from build123d import *

# Parameters (mm, degrees)
F0_W           = 30
F0_H           = 30
F0_R           = 4
F1_DEPTH       = 11
F3_D           = 3.4
F3_CBORE_D     = 6.3
F3_CBORE_DEPTH = 8.5
F5_D           = 3.4
F6_DEPTH       = 5
F7_R           = 4
F8_DEPTH       = 7
F9_R           = 5
F10_T1_DEPTH   = 9.5
F10_T3_DEPTH   = 20
F10_T5_DEPTH   = 20
F10_T12_ANGLE  = 90
F10_T14_ANGLE  = 90
F10_T16_ANGLE  = 90
F10_T18_ANGLE  = 90


# Not quite as in the source:
# - a fillet or chamfer that OpenCascade refuses, or shapes differently, is made with other operations: its cross-section is extruded or revolved along the edge and cut away or added


with BuildPart() as f1:
    # F0 (on Top) → F1 (new body)
    with BuildSketch(Plane.XY):
        Rectangle(F0_W, F0_H)
        Circle(F0_R, mode=Mode.SUBTRACT)
    extrude(amount=F1_DEPTH)

    # F3 (through all)
    with Locations(Plane.XY.offset(11)):
        with Locations((-6.7175144213, -6.7175144213), (-5.6568542495, 5.6568542495), (6.7175144213, 6.7175144213), (5.6568542495, -5.6568542495)):
            CounterBoreHole(F3_D / 2, F3_CBORE_D / 2, F3_CBORE_DEPTH)

    # F5 (through all)
    with Locations(Plane(origin=(0, 0, 0), x_dir=(1, 0, 0), z_dir=(0, 0, -1))):
        with Locations((-11, 0), (11, 0)):
            Hole(F5_D / 2)

    # F4 (on face) → F6 (cut)
    with BuildSketch(Plane(origin=(0, 0, 0), x_dir=(1, 0, 0), z_dir=(0, 0, -1))):
        Polygon((14, -1.7320508076), (14, 1.7320508076), (11, 3.4641016151), (8, 1.7320508076), (8, -1.7320508076), (11, -3.4641016151), align=None)
        Polygon((-8, -1.7320508076), (-8, 1.7320508076), (-11, 3.4641016151), (-14, 1.7320508076), (-14, -1.7320508076), (-11, -3.4641016151), align=None)
    extrude(amount=-F6_DEPTH, mode=Mode.SUBTRACT)

    # F7 (on face) → F8 (cut)
    with BuildSketch(Plane.XY.offset(11)):
        with BuildLine():
            Line((-7.75, -15), (7.75, -15))
            Line((7.75, -15), (7.75, -8.0108382909))
            ThreePointArc((7.75, -8.0108382909), (2.5068542495, -5.6568542495), (7.75, -3.3028702081))
            Line((7.75, -3.3028702081), (7.75, 3.7415316374))
            ThreePointArc((7.75, 3.7415316374), (3.5675144213, 6.7175144213), (7.75, 9.6934972051))
            Line((7.75, 9.6934972051), (7.75, 15))
            Line((7.75, 15), (-7.75, 15))
            Line((-7.75, 15), (-7.75, 8.0108382909))
            ThreePointArc((-7.75, 8.0108382909), (-4.3666816087, 8.5305199498), (-2.5068542495, 5.6568542495))
            ThreePointArc((-2.5068542495, 5.6568542495), (-4.3666816087, 2.7831885492), (-7.75, 3.3028702081))
            Line((-7.75, 3.3028702081), (-7.75, -3.7415316374))
            ThreePointArc((-7.75, -3.7415316374), (-4.8912928538, -4.1509184682), (-3.5675144213, -6.7175144213))
            ThreePointArc((-3.5675144213, -6.7175144213), (-4.8912928538, -9.2841103744), (-7.75, -9.6934972051))
            Line((-7.75, -9.6934972051), (-7.75, -15))
        make_face()
        Circle(F7_R, mode=Mode.SUBTRACT)
    extrude(amount=-F8_DEPTH, mode=Mode.SUBTRACT)

    # F9
    f9_edges = [f1.edges().sort_by_distance(p)[0] for p in [
        (15, 15, 5.5),
        (-15, 15, 5.5),
        (15, -15, 5.5),
        (-15, -15, 5.5),
    ]]
    fillet(f9_edges, radius=F9_R)

    # F10: fillet of radius 1 on 15 edges, made by hand

    # F10_s2 → F10_t1 (cut)
    with BuildSketch(Plane.XY.offset(4)):
        with BuildLine():
            ThreePointArc((8.75, 15), (8.0428932188, 14.7071067812), (7.75, 14))
            Line((7.75, 14), (7.75, 15))
            Line((7.75, 15), (8.75, 15))
        make_face()
        with BuildLine():
            ThreePointArc((-8.75, 15), (-8.0428932188, 14.7071067812), (-7.75, 14))
            Line((-7.75, 14), (-7.75, 15))
            Line((-7.75, 15), (-8.75, 15))
        make_face()
        with BuildLine():
            ThreePointArc((8.75, -15), (8.0428932188, -14.7071067812), (7.75, -14))
            Line((7.75, -14), (7.75, -15))
            Line((7.75, -15), (8.75, -15))
        make_face()
        with BuildLine():
            ThreePointArc((-8.75, -15), (-8.0428932188, -14.7071067812), (-7.75, -14))
            Line((-7.75, -14), (-7.75, -15))
            Line((-7.75, -15), (-8.75, -15))
        make_face()
    extrude(amount=F10_T1_DEPTH, mode=Mode.SUBTRACT)

    # F10_s4 → F10_t3 (cut)
    with BuildSketch(Plane.YZ.offset(-10)):
        with BuildLine():
            ThreePointArc((-15, 1), (-14.7071067812, 0.2928932188), (-14, 0))
            Line((-14, 0), (-15, 0))
            Line((-15, 0), (-15, 1))
        make_face()
        with BuildLine():
            ThreePointArc((14, 0), (14.7071067812, 0.2928932188), (15, 1))
            Line((15, 1), (15, 0))
            Line((15, 0), (14, 0))
        make_face()
    extrude(amount=F10_T3_DEPTH, mode=Mode.SUBTRACT)

    # F10_s6 → F10_t5 (cut)
    with BuildSketch(Plane.XZ.offset(-10)):
        with BuildLine():
            ThreePointArc((-14, 0), (-14.7071067812, 0.2928932188), (-15, 1))
            Line((-15, 1), (-15, 0))
            Line((-15, 0), (-14, 0))
        make_face()
        with BuildLine():
            ThreePointArc((14, 0), (14.7071067812, 0.2928932188), (15, 1))
            Line((15, 1), (15, 0))
            Line((15, 0), (14, 0))
        make_face()
    extrude(amount=F10_T5_DEPTH, mode=Mode.SUBTRACT)

    # F10_s7 → F10_t8 (revolve, cut)
    with BuildSketch(Plane.XZ):
        with BuildLine():
            ThreePointArc((5, 4), (4.2928932188, 3.7071067812), (4, 3))
            Line((4, 3), (4, 4))
            Line((4, 4), (5, 4))
        make_face()
    revolve(axis=Axis((0, 0, 4), (0, 0, 1)), mode=Mode.SUBTRACT)

    # F10_s9 → F10_t10 (revolve, cut)
    with BuildSketch(Plane.XZ):
        with BuildLine():
            ThreePointArc((5, 0), (4.2928932188, 0.2928932188), (4, 1))
            Line((4, 1), (4, 0))
            Line((4, 0), (5, 0))
        make_face()
    revolve(axis=Axis((0, 0, 0), (0, 0, 1)), mode=Mode.SUBTRACT)

    # F10_s11 → F10_t12 (revolve, cut)
    with BuildSketch(Plane.YZ.offset(-10)):
        with BuildLine():
            ThreePointArc((-14, 0), (-14.7071067812, 0.2928932188), (-15, 1))
            Line((-15, 1), (-15, 0))
            Line((-15, 0), (-14, 0))
        make_face()
    revolve(axis=Axis((-10, -10, 0), (0, 0, -1)), revolution_arc=F10_T12_ANGLE, mode=Mode.SUBTRACT)

    # F10_s13 → F10_t14 (revolve, cut)
    with BuildSketch(Plane.YZ.offset(10)):
        with BuildLine():
            ThreePointArc((-14, 0), (-14.7071067812, 0.2928932188), (-15, 1))
            Line((-15, 1), (-15, 0))
            Line((-15, 0), (-14, 0))
        make_face()
    revolve(axis=Axis((10, -10, 0), (0, 0, 1)), revolution_arc=F10_T14_ANGLE, mode=Mode.SUBTRACT)

    # F10_s15 → F10_t16 (revolve, cut)
    with BuildSketch(Plane.XZ.offset(-10)):
        with BuildLine():
            ThreePointArc((-14, 0), (-14.7071067812, 0.2928932188), (-15, 1))
            Line((-15, 1), (-15, 0))
            Line((-15, 0), (-14, 0))
        make_face()
    revolve(axis=Axis((-10, 10, 0), (0, 0, -1)), revolution_arc=F10_T16_ANGLE, mode=Mode.SUBTRACT)

    # F10_s17 → F10_t18 (revolve, cut)
    with BuildSketch(Plane.XZ.offset(-10)):
        with BuildLine():
            ThreePointArc((14, 0), (14.7071067812, 0.2928932188), (15, 1))
            Line((15, 1), (15, 0))
            Line((15, 0), (14, 0))
        make_face()
    revolve(axis=Axis((10, 10, 0), (0, 0, 1)), revolution_arc=F10_T18_ANGLE, mode=Mode.SUBTRACT)


solid = f1.part
Could you check a few things on this model? Use its own coordinates, in mm. A direction names the side the tool comes from. Coordinates: 2 decimals unless noted, no trailing zeros. Order: outer loops, then holes, each group sorted by start corner. A loop starts at its lowest first (then second) coordinate and runs counter-clockwise, first axis right, second up. Notation, with made-up numbers: (76.25, -17) - (128.25, -17) arc R28 cw to (128.25, 6) - close; hole circle Ø6 at (16.5, 52.5). An arc over 180 degrees is marked (long way). Answer in a Markdown table with one row per item. Add a question column.
(1) I need wall thicknesses on L1, parallel to Y at x = 0, z = 1.8; L2, parallel to X at y = 9.75, z = 7.5; L3, parallel to Y at x = -2, z = 2.5. Which ranges of each line are inside material? Lowest first, please.
(2) Will these pins go through, and if not, where does the flat tip stop? pin 1 (2.5 mm diameter, centred on x = -5.66, y = 5.66, fed in from -Z); pin 2 (4.5 mm diameter, centred on x = 5.66, y = -5.66, fed in from +Z); pin 3 (1.8 mm diameter, centred on x = 12.5, y = 0.5, fed in from -Z); pin 4 (2 mm diameter, centred on y = -12.5, z = 7, fed in from +X).
(3) If we section it at A-A, the plane z = 6.5: Please give me the cut outline in (x, y), then the cut area to 3 significant figures.
(4) If we mould it in two halves opening along X, with no side actions, what happens to faces 4 (the face through (9.43, 0.65, 8.04)), 5 (the face through (13, 14, 6)), 6 (the face through (-9.5, -2.6, 2.5)), 7 (the face through (-0.14, 14.699, 0.285))? For each: released by +X, released by -X, zero draft, split by the parting line, or undercut.
(5) If we section it at C-C, the plane y = 0: State how many separate pieces and enclosed holes the cut face has, then the cut area to 3 significant figures.
(6) On a 3-axis mill with a long thin cutter (end or side, diameter ignored), from which of +Z, -Z, +X, -X, +Y, -Y can I reach the whole of each face in a straight line? I mean faces 1 (the face through (9.627, 5.511, 5.865)), 2 (the face through (-7.75, 11, 8)), 3 (the face through (14, 0, 2)). Say none if no direction works.
(7) If we section it at B-B, the plane x = 0: Please give me the cut outline in (y, z).
Results are:
| question | item | result |
|---|---|---|
| 1 | L1 | y = -15 to -4, 4 to 15 |
| 1 | L2 | x = -15 to -7.75, 7.75 to 15 |
| 1 | L3 | y = -15 to -3.46, 3.46 to 15 |
| 2 | pin 1 | passes through |
| 2 | pin 2 | stops at z = 2.5 |
| 2 | pin 3 | stops at z = 5 |
| 2 | pin 4 | stops at x = 14.77 |
| 3 | outline | (-15, -10) arc R5 ccw to (-10, -15) - (-8.75, -15) arc R1 ccw to (-7.75, -14) - (-7.75, -9.69) arc R3.15 cw to (-7.75, -3.74) - (-7.75, 3.3) arc R3.15 cw to (-7.75, 8.01) - (-7.75, 14) arc R1 ccw to (-8.75, 15) - (-10, 15) arc R5 ccw to (-15, 10) - close; (7.75, -14) arc R1 ccw to (8.75, -15) - (10, -15) arc R5 ccw to (15, -10) - (15, 10) arc R5 ccw to (10, 15) - (8.75, 15) arc R1 ccw to (7.75, 14) - (7.75, 9.69) arc R3.15 cw to (7.75, 3.74) - (7.75, -3.3) arc R3.15 cw to (7.75, -8.01) - close; hole circle Ø3.4 at (-11, 0); hole circle Ø3.4 at (11, 0) |
| 3 | area | 369 mm2 |
| 4 | face 4 | undercut |
| 4 | face 5 | released by +X |
| 4 | face 6 | undercut |
| 4 | face 7 | zero draft |
| 5 | separate pieces | 4 |
| 5 | enclosed holes | 0 |
| 5 | area | 87.4 mm2 |
| 6 | face 1 | +Z |
| 6 | face 2 | +Z, +Y, -Y |
| 6 | face 3 | -Z |
| 7 | outline | (-15, 1) arc R1 ccw to (-14, 0) - (-5, 0) arc R1 ccw to (-4, 1) - (-4, 3) arc R1 ccw to (-5, 4) - (-15, 4) - close; (4, 1) arc R1 ccw to (5, 0) - (14, 0) arc R1 ccw to (15, 1) - (15, 4) - (5, 4) arc R1 ccw to (4, 3) - close |
